Part model, mm, in its own coordinate system. Face numbers are marked on the shaded views. A direction names the side the tool comes from. Round coordinates to 2 decimals unless told otherwise and drop trailing zeros. Loops run counter-clockwise (first coordinate to the right, second up) from the corner with the lowest first, then second, coordinate; pieces in that order, holes last. Notation, with made-up numbers: (20, -0.75) -> (59, -0.75) arc R4 ccw to (59, 4.25) -> close; hole circle Ø10 at (83, 54.25). An arc over 180 degrees is marked (long way). Use a Markdown table: item, result. Add a question column.
Item 1: Cut at C-C, the plane y = 10.5. List the corners of the cut face in (x, z), plus the area to 3 significant figures.
Item 2: Probe line 1 (Z direction, x = 41.5, y = 6.5); line 2 (X direction, y = 47, z = 110); line 3 (X direction, y = 3.5, z = 54.5). List the from-to ranges inside material, lowest first. Write a range as [from, to].
Item 3: Flat gauge pins, fed straight in: pin 1 (8 mm diameter, centred on x = 68.5, y = 35, fed in from -Z); pin 2 (5 mm diameter, centred on y = 36, z = 16, fed in from -X); pin 3 (1 mm diameter, centred on x = 70.5, y = 17.5, fed in from +Z); pin 4 (12.5 mm diameter, centred on y = 18.5, z = 86.5, fed in from -X). Where does each tip first touch, or does it go through?
Item 4: Cut at B-B, the plane x = 33. List the corners of the cut face in (y, z), plus the area to 3 significant figures.
Item 5: Which spindle directions (+Z, -Z, +X, -X, +Y, -Y) get a long thin tool onto all of the face, cutting with end or side? Do the marked faces 1, 2 and 3. Say none if no direction does.
Item 6: Cut at A-A, the plane y = 40. List the corners of the cut face in (x, z), plus the area to 3 significant figures.
Item 7: Cut at D-D, the plane z = 58. List the corners of the cut face in (x, y).
```python
from build123d import *

# Parameters (mm, degrees)
BOSS_EXTRUDE1_DEPTH = 50
FILLET1_R           = 5
CUT_EXTRUDE1_DEPTH  = 3
CUT_EXTRUDE2_DEPTH  = 3
FILLET2_R           = 5


with BuildPart() as part:
    # Sketch1 → Boss-Extrude1 (new body)
    with BuildSketch(Plane(origin=(0, 0, 0), x_dir=(1, 0, 0), z_dir=(0, 1, 0))):
        Polygon((0, 0), (0, -65), (79, -65), (79, -115), (76, -115), (76, -68), (-3, -68), (-3, 0), align=None)
    extrude(amount=BOSS_EXTRUDE1_DEPTH)

    # Fillet1
    fillet1_edges = [part.edges().sort_by_distance(p)[0] for p in [
        (0, 25, 65),
        (79, 25, 65),
        (76, 25, 68),
        (-3, 25, 68),
    ]]
    fillet(fillet1_edges, radius=FILLET1_R)

    # Sketch2 → Cut-Extrude1 (cut)
    with BuildSketch(Plane.ZY.offset(-76)):
        with BuildLine():
            Line((87.5, 45), (102.5, 45))
            ThreePointArc((102.5, 45), (107.5, 40), (102.5, 35))
            Line((102.5, 35), (87.5, 35))
            ThreePointArc((87.5, 35), (82.5, 40), (87.5, 45))
        make_face()
        with BuildLine():
            Line((87.5, 15), (102.5, 15))
            ThreePointArc((102.5, 15), (107.5, 10), (102.5, 5))
            Line((102.5, 5), (87.5, 5))
            ThreePointArc((87.5, 5), (82.5, 10), (87.5, 15))
        make_face()
    extrude(amount=-CUT_EXTRUDE1_DEPTH, mode=Mode.SUBTRACT)

    # Sketch3 → Cut-Extrude2 (cut)
    with BuildSketch(Plane.ZY.offset(3)):
        with BuildLine():
            Line((12.5, 45), (27.5, 45))
            ThreePointArc((27.5, 45), (32.5, 40), (27.5, 35))
            Line((27.5, 35), (12.5, 35))
            ThreePointArc((12.5, 35), (7.5, 40), (12.5, 45))
        make_face()
        with BuildLine():
            Line((12.5, 15), (27.5, 15))
            ThreePointArc((27.5, 15), (32.5, 10), (27.5, 5))
            Line((27.5, 5), (12.5, 5))
            ThreePointArc((12.5, 5), (7.5, 10), (12.5, 15))
        make_face()
    extrude(amount=-CUT_EXTRUDE2_DEPTH, mode=Mode.SUBTRACT)

    # Fillet2
    fillet2_edges = [part.edges().sort_by_distance(p)[0] for p in [
        (-1.5, 0, 0),
        (77.5, 50, 115),
        (-1.5, 50, 0),
        (77.5, 0, 115),
    ]]
    fillet(fillet2_edges, radius=FILLET2_R)


solid = part.part
```
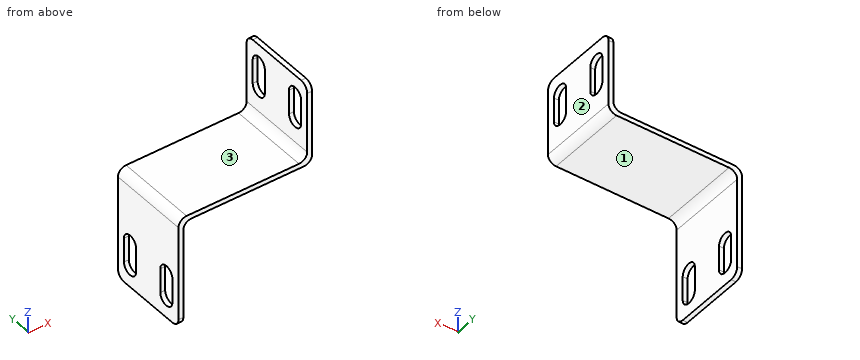
A:
| question | item | result |
|---|---|---|
| 1 | outline | (-3, 0) -> (0, 0) -> (0, 7.53) -> (-3, 7.53) -> close; (-3, 32.47) -> (0, 32.47) -> (0, 60) arc R5 cw to (5, 65) -> (74, 65) arc R5 ccw to (79, 70) -> (79, 82.53) -> (76, 82.53) -> (76, 73) arc R5 cw to (71, 68) -> (2, 68) arc R5 ccw to (-3, 63) -> close; (76, 107.47) -> (79, 107.47) -> (79, 115) -> (76, 115) -> close |
| 1 | area | 432 mm^2 |
| 2 | line 1 | z = [65, 68] |
| 2 | line 2 | x = [76, 79] |
| 2 | line 3 | x = [-3, 0] |
| 3 | pin 1 | stops at z = 65 |
| 3 | pin 2 | stops at x = -3 |
| 3 | pin 3 | stops at z = 68 |
| 3 | pin 4 | stops at x = 76 |
| 4 | outline | (0, 65) -> (50, 65) -> (50, 68) -> (0, 68) -> close |
| 4 | area | 150 mm^2 |
| 5 | face 1 | -Z, +X, +Y, -Y |
| 5 | face 2 | +Z, -Z, +X, +Y, -Y |
| 5 | face 3 | +Z, -X, +Y, -Y |
| 6 | outline | (-3, 0) -> (0, 0) -> (0, 7.5) -> (-3, 7.5) -> close; (-3, 32.5) -> (0, 32.5) -> (0, 60) arc R5 cw to (5, 65) -> (74, 65) arc R5 ccw to (79, 70) -> (79, 82.5) -> (76, 82.5) -> (76, 73) arc R5 cw to (71, 68) -> (2, 68) arc R5 ccw to (-3, 63) -> close; (76, 107.5) -> (79, 107.5) -> (79, 115) -> (76, 115) -> close |
| 6 | area | 432 mm^2 |
| 7 | outline | (-3, 0) -> (0, 0) -> (0, 50) -> (-3, 50) -> close |
